```python
from build123d import *

# Parameters (mm, degrees)
SKETCH1_R           = 1.5
BOSS_EXTRUDE1_DEPTH = 3
BOSS_EXTRUDE2_DEPTH = 25
SKETCH6_W           = 56
SKETCH6_H           = 9.11547301
CUT_EXTRUDE1_DEPTH  = 63.91555103
FILLET1_R           = 2
FILLET2_R           = 1
BOSS_EXTRUDE4_DEPTH = 2.460910909
BOSS_EXTRUDE5_DEPTH = 56
FILLET3_R           = 1


with BuildPart() as part:
    # Sketch1 → Boss-Extrude1 (new body)
    with BuildSketch(Plane.XY):
        with BuildLine():
            ThreePointArc((2.68220241, -18.5), (2.975095629, -19.207106781), (3.68220241, -19.5))
            Line((3.68220241, -19.5), (18.54616344, -19.5))
            ThreePointArc((18.54616344, -19.5), (19.008103207, -19.191341716), (18.899716831, -18.646446609))
            Line((18.899716831, -18.646446609), (15.000000504, -14.746730282))
            Line((15.000000504, -14.746730282), (2.601508845, -2.348238623))
            Line((2.601508845, -2.348238623), (1.894402064, -1.641131842))
            Line((1.894402064, -1.641131842), (2.601508845, -0.934025061))
            Line((2.601508845, -0.934025061), (2.927422074, -0.608111832))
            Line((2.927422074, -0.608111832), (3.634528855, 0.098994949))
            Line((3.634528855, 0.098994949), (2.927422074, 0.806101731))
            Line((2.927422074, 0.806101731), (0.806101731, 2.927422074))
            ThreePointArc((0.806101731, 2.927422074), (0.098994949, 3.220315293), (-0.608111832, 2.927422074))
            Line((-0.608111832, 2.927422074), (-1.641131842, 1.894402064))
            Line((-1.641131842, 1.894402064), (-3.762452186, -0.22691828))
            ThreePointArc((-3.762452186, -0.22691828), (-4.348238623, -1.641131842), (-3.762452186, -3.055345405))
            Line((-3.762452186, -3.055345405), (1.803522753, -8.621320344))
            ThreePointArc((1.803522753, -8.621320344), (2.453841007, -9.59459039), (2.68220241, -10.742640687))
            Line((2.68220241, -10.742640687), (2.68220241, -18.5))
        make_face()
        Circle(SKETCH1_R, mode=Mode.SUBTRACT)
    boss_extrude1 = extrude(amount=BOSS_EXTRUDE1_DEPTH)

    # Sketch2 → Boss-Extrude2 (add)
    with BuildSketch(Plane.XY.offset(3)):
        with BuildLine():
            Line((18.899716831, -18.646446609), (10.995910909, -10.742640687))
            Line((10.995910909, -10.742640687), (2.68220241, -10.742640687))
            Line((2.68220241, -10.742640687), (2.68220241, -18.5))
            ThreePointArc((2.68220241, -18.5), (2.975095629, -19.207106781), (3.68220241, -19.5))
            Line((3.68220241, -19.5), (18.54616344, -19.5))
            ThreePointArc((18.54616344, -19.5), (19.008103207, -19.191341716), (18.899716831, -18.646446609))
        make_face()
    boss_extrude2 = extrude(amount=BOSS_EXTRUDE2_DEPTH)

    # Mirror1: Boss-Extrude1, Boss-Extrude2 across plane
    add(boss_extrude1.mirror(Plane.XY.offset(28)))
    add(boss_extrude2.mirror(Plane.XY.offset(28)))

    # Sketch6 → Cut-Extrude1 (cut, through all)
    with BuildSketch(Plane(origin=(-6.530219139, -6.530219139, 0), x_dir=(0, 0, 1), z_dir=(-0.7071067811865487, -0.7071067811865465, 0))):
        with Locations((28, -17.586068001)):
            Rectangle(SKETCH6_W, SKETCH6_H)
    extrude(amount=CUT_EXTRUDE1_DEPTH, mode=Mode.SUBTRACT)

    # Fillet1
    fillet1_edges = [part.edges().sort_by_distance(p)[0] for p in [
        (6.439561723, -19.5, 28),
    ]]
    fillet(fillet1_edges, radius=FILLET1_R)

    # Fillet2
    fillet2_edges = [part.edges().sort_by_distance(p)[0] for p in [
        (2.68220241, -15.742640687, 28),
    ]]
    fillet(fillet2_edges, radius=FILLET2_R)

    # Sketch9 → Boss-Extrude4 (add)
    with BuildSketch(Plane(origin=(0.126635111, 0.126635111, 0), x_dir=(0, 0, -1), z_dir=(0.7071067811865487, 0.7071067811865465, 0))):
        Polygon((-56, -2.5), (-53, -2.5), (-53, -15.371477247), (-3, -15.371477247), (-3, -2.5), (0, -2.5), (0, -26.549146776), (-56, -26.549146776), align=None)
    extrude(amount=BOSS_EXTRUDE4_DEPTH)

    # Sketch10 → Boss-Extrude5 (add)
    with BuildSketch(Plane(origin=(0, 0, 0), x_dir=(-1, 0, 0), z_dir=(0, 0, -1))):
        Polygon((-20.639843623, -16.906319818), (-18.04616344, -19.5), (-23.233523805, -19.5), align=None)
    extrude(amount=-BOSS_EXTRUDE5_DEPTH)

    # Fillet3
    fillet3_edges = [part.edges().sort_by_distance(p)[0] for p in [
        (23.233523805, -19.5, 28),
    ]]
    fillet(fillet3_edges, radius=FILLET3_R)


solid = part.part
```
The listing builds one solid part. Answer for the finished solid, in the listing's coordinates (mm). A direction names the side the tool comes from. Give positions to 0.01 mm unless a question says otherwise; leave off trailing zeros. Order: outer loops, then holes, each group sorted by start corner. A loop starts at its lowest first (then second) coordinate and runs counter-clockwise, first axis right, second up. Notation, with made-up numbers: (-9, 66.5) -> (40, 66.5) arc R27 cw to (40, 104.5) -> close; hole circle Ø10 at (-38.5, 5). An arc over 180 degrees is marked (long way). Answer as CSV lines item,"result". Start each with the question number.
Q1. A cutting plane is placed at B-B (x = 0). Determine the outline of the cut face in (y, z).
Q2. A cutting plane is placed at A-A (z = 49). Determine the outline of the cut face in (x, y), then the cut area to 3 significant figures.
Q3. Determine the mould class of faces 3 (the cylindrical face through (21.737, -18.898, 28.392)), 4 (the cylindrical face through (-1.5, 0.07, 1.48)), 5 (the flat face through (2.682, -13, 28)) for opening direction X: pulls with the +X half, pulls with the -X half, needs draft (parallel to the pull), parting line crosses it, or undercut.
Q4. Given pin 1 (8 mm diameter, centred on x = 1.5, z = 20, fed in from -Y); pin 2 (10 mm diameter, centred on x = 17, y = -9, fed in from +Z); pin 3 (12 mm diameter, centred on y = -9, z = 16.5, fed in from -X); pin 4 (2 mm diameter, centred on x = 10, y = -2.5, fed in from +Z), each flat-ended and moving along its own axis, determine where each tip first touches the part or whether it passes through.
Q5. A cutting plane is placed at D-D (y = -12). Determine the outline of the cut face in (x, z).
Q6. Find the intervals of material crossed by L1, parallel to Z at x = 3.25, y = -6.5; L2, parallel to Y at x = 7.75, z = 47.5; L3, parallel to Y at x = 0, z = 2.2, in increasing order.
Q7. A cutting plane is placed at C-C (x = 8). Determine the outline of the cut face in (y, z), then the cut area to 3 significant figures.
Q8. Which of the six approach directions +Z, -Z, +X, -X, +Y, -Y give full straight-line access (tool end or side, diameter ignored) to faces 1 (the flat face through (4, -5, 53)), 2 (the flat face through (4.39, -17.45, 27.61))?
Results found:
1,outline,"(-6.82, 0) -> (-1.5, 0) -> (-1.5, 3) -> (-6.82, 3) -> close; (-6.82, 53) -> (-1.5, 53) -> (-1.5, 56) -> (-6.82, 56) -> close; (1.5, 0) -> (3.22, 0) -> (3.22, 3) -> (1.5, 3) -> close; (1.5, 53) -> (3.22, 53) -> (3.22, 56) -> (1.5, 56) -> close"
2,outline,"(2.68, -15.33) arc R1 ccw to (2.98, -16.04) -> (5.85, -18.91) arc R2 ccw to (7.27, -19.5) -> (20.82, -19.5) arc R1 ccw to (21.53, -17.79) -> (12.74, -9) -> (11, -10.74) -> (2.68, -10.74) -> close"
2,area,"136 mm2"
3,face 3,"pulls with the +X half"
3,face 4,"undercut"
3,face 5,"pulls with the -X half"
4,pin 1,"y = -18.56"
4,pin 2,"z = 56"
4,pin 3,"x = 2.68"
4,pin 4,"through"
5,outline,"(2.68, 0) -> (15.73, 0) -> (15.73, 56) -> (2.68, 56) -> close"
6,L1,"0 to 3, 53 to 56"
6,L2,"-19.5 to -10.74"
6,L3,"-6.82 to -1.5, 1.5 to 3.22"
7,outline,"(-19.5, 0) -> (-4.27, 0) -> (-4.27, 3) -> (-10.74, 3) -> (-10.74, 53) -> (-4.27, 53) -> (-4.27, 56) -> (-19.5, 56) -> close"
7,area,"529 mm2"
8,face 1,"-X, +Y"
8,face 2,"+Z, -Z, -X, -Y"
